from build123d import *

# Parameters (mm, degrees)
CROQUIS2_R                  = 4.1
SALIENTE_EXTRUIR1_DEPTH     = 35
CROQUIS3_W                  = 24
CROQUIS3_H                  = 12.1
CORTAR_EXTRUIR1_DEPTH       = 24
CROQUIS9_R                  = 1.7
CORTAR_EXTRUIR2_DEPTH       = 10
CORTAR_EXTRUIR3_START       = -10
CROQUIS11_R                 = 25
CORTAR_EXTRUIR3_DEPTH       = 10
CORTAR_EXTRUIR5_START       = 13.655231177
CORTAR_EXTRUIR5_DEPTH       = 8
CORTAR_EXTRUIR5_START_2     = 6.155231177
CORTAR_EXTRUIR5_2_DEPTH     = 5
CORTAR_EXTRUIR5_START_3     = 24.155231177
CORTAR_EXTRUIR5_3_DEPTH     = 5
CORTAR_EXTRUIR6_START       = -10
CROQUIS13_R                 = 25
CORTAR_EXTRUIR6_DEPTH       = 10
CROQUIS14_R                 = 11.035
CORTAR_EXTRUIR7_DEPTH       = 8.05
CORTAR_EXTRUIR8_DEPTH       = 15
CORTAR_EXTRUIR8_DEPTH_BACK  = 7
CORTAR_EXTRUIR9_DEPTH       = 15
CORTAR_EXTRUIR9_DEPTH_BACK  = 7
CORTAR_EXTRUIR10_DEPTH      = 15
CORTAR_EXTRUIR10_DEPTH_BACK = 7
CORTAR_EXTRUIR11_DEPTH      = 121.441894704
REDONDEO1_R                 = 30
CROQUIS22_W                 = 11.434183309
CROQUIS22_H                 = 8.348024574
CORTAR_EXTRUIR12_DEPTH      = 10


# Read off the part's stored shape, not the designer's step: Cortar-Extruir5
with BuildPart() as part:
    # Croquis2 → Saliente-Extruir1 (new body)
    with BuildSketch(Plane.XY):
        with BuildLine():
            Line((-11.5, 104.898979486), (-21.7, 104.898979486))
            Line((-21.7, 104.898979486), (-21.7, 100.380604651))
            Line((-21.7, 100.380604651), (-12.49420426, 100.380604651))
            ThreePointArc((-12.49420426, 100.380604651), (-12.498149406, 99.784915281), (-12.473709842, 99.189714392))
            ThreePointArc((-12.473709842, 99.189714392), (-16.573234399, 52.954310766), (-23.961892015, 7.129356989))
            ThreePointArc((-23.961892015, 7.129356989), (0, -25), (23.961892015, 7.129356989))
            ThreePointArc((23.961892015, 7.129356989), (16.547311175, 52.357383104), (12.33822575, 97.995458822))
            ThreePointArc((12.33822575, 97.995458822), (12.473356614, 99.184294915), (12.49420426, 100.380604651))
            Line((12.49420426, 100.380604651), (21.7, 100.380604651))
            Line((21.7, 100.380604651), (21.7, 104.898979486))
            Line((21.7, 104.898979486), (11.5, 104.898979486))
            ThreePointArc((11.5, 104.898979486), (0, 112.5), (-11.5, 104.898979486))
        make_face()
        Circle(CROQUIS2_R, mode=Mode.SUBTRACT)
    extrude(amount=SALIENTE_EXTRUIR1_DEPTH)

    # Croquis3 → Cortar-Extruir1 (cut)
    with BuildSketch(Plane(origin=(0, 112.5, 0), x_dir=(1, 0, 0), z_dir=(0, 1, 0))):
        with Locations((0, -17.5)):
            Rectangle(CROQUIS3_W, CROQUIS3_H)
    extrude(amount=-CORTAR_EXTRUIR1_DEPTH, mode=Mode.SUBTRACT)

    # Croquis9 → Cortar-Extruir2 (cut)
    with BuildSketch(Plane(origin=(0, 104.898979486, 0), x_dir=(1, 0, 0), z_dir=(0, 1, 0))):
        with Locations(Location((-15.2, -17.5, 0), (0, 0, 270))):
            Circle(CROQUIS9_R)
        with Locations(Location((15.2, -17.5, 0), (0, 0, 270))):
            Circle(CROQUIS9_R)
    extrude(amount=-CORTAR_EXTRUIR2_DEPTH, mode=Mode.SUBTRACT)

    # Croquis11 → Cortar-Extruir3 (cut)
    with BuildSketch(Plane.XY.offset(35).offset(CORTAR_EXTRUIR3_START)):
        Circle(CROQUIS11_R)
    extrude(amount=CORTAR_EXTRUIR3_DEPTH, mode=Mode.SUBTRACT)

    # Cortar-Extruir5 outline → Cortar-Extruir5 (cut)
    with BuildSketch(Plane.XY.offset(CORTAR_EXTRUIR5_START)):
        with BuildLine():
            Line((12.387970466, 97.129356989), (12, 97.129356989))
            Line((12, 97.129356989), (12, 88.5))
            Line((12, 88.5), (7.946995801, 88.5))
            ThreePointArc((7.946995801, 88.5), (12.16824242, 47.640569315), (18.961892015, 7.129356989))
            Line((18.961892015, 7.129356989), (23.961892015, 7.129356989))
            ThreePointArc((23.961892015, 7.129356989), (16.602493766, 51.9271429), (12.387970466, 97.129356989))
        make_face()
    extrude(amount=CORTAR_EXTRUIR5_DEPTH, mode=Mode.SUBTRACT)

    # Cortar-Extruir5 2 outline → Cortar-Extruir5 2 (cut)
    with BuildSketch(Plane.XY.offset(CORTAR_EXTRUIR5_START_2)):
        with BuildLine():
            ThreePointArc((12.902326037, 89.129356989), (12.63281503, 93.128564031), (12.387970466, 97.129356989))
            Line((12.387970466, 97.129356989), (7.387970466, 97.129356989))
            ThreePointArc((7.387970466, 97.129356989), (7.63281503, 93.128564031), (7.902326037, 89.129356989))
            Line((7.902326037, 89.129356989), (12.902326037, 89.129356989))
        make_face()
        with BuildLine():
            ThreePointArc((15.954808066, 57.129356989), (15.485901101, 61.127943182), (15.041769556, 65.129356989))
            Line((15.041769556, 65.129356989), (10.041769556, 65.129356989))
            ThreePointArc((10.041769556, 65.129356989), (10.485901101, 61.127943182), (10.954808066, 57.129356989))
            Line((10.954808066, 57.129356989), (15.954808066, 57.129356989))
        make_face()
        with BuildLine():
            ThreePointArc((18.985918027, 35.129356989), (18.378022509, 39.127504621), (17.795013863, 43.129356989))
            Line((17.795013863, 43.129356989), (12.795013863, 43.129356989))
            ThreePointArc((12.795013863, 43.129356989), (13.378022509, 39.127504621), (13.985918027, 35.129356989))
            Line((13.985918027, 35.129356989), (18.985918027, 35.129356989))
        make_face()
    extrude(amount=CORTAR_EXTRUIR5_2_DEPTH, mode=Mode.SUBTRACT)

    # Cortar-Extruir5 3 outline → Cortar-Extruir5 3 (cut)
    with BuildSketch(Plane.XY.offset(CORTAR_EXTRUIR5_START_3)):
        with BuildLine():
            ThreePointArc((13.684802762, 79.129356989), (13.35325681, 83.128371707), (13.046404729, 87.129356989))
            Line((13.046404729, 87.129356989), (8.046404729, 87.129356989))
            ThreePointArc((8.046404729, 87.129356989), (8.35325681, 83.128371707), (8.684802762, 79.129356989))
            Line((8.684802762, 79.129356989), (13.684802762, 79.129356989))
        make_face()
        with BuildLine():
            ThreePointArc((15.954808066, 57.129356989), (15.485901101, 61.127943182), (15.041769556, 65.129356989))
            Line((15.041769556, 65.129356989), (10.041769556, 65.129356989))
            ThreePointArc((10.041769556, 65.129356989), (10.485901101, 61.127943182), (10.954808066, 57.129356989))
            Line((10.954808066, 57.129356989), (15.954808066, 57.129356989))
        make_face()
        with BuildLine():
            ThreePointArc((18.985918027, 35.129356989), (18.378022509, 39.127504621), (17.795013863, 43.129356989))
            Line((17.795013863, 43.129356989), (12.795013863, 43.129356989))
            ThreePointArc((12.795013863, 43.129356989), (13.378022509, 39.127504621), (13.985918027, 35.129356989))
            Line((13.985918027, 35.129356989), (18.985918027, 35.129356989))
        make_face()
    extrude(amount=CORTAR_EXTRUIR5_3_DEPTH, mode=Mode.SUBTRACT)

    # Croquis13 → Cortar-Extruir6 (cut)
    with BuildSketch(Plane.XY.offset(25).offset(CORTAR_EXTRUIR6_START)):
        Circle(CROQUIS13_R)
    extrude(amount=CORTAR_EXTRUIR6_DEPTH, mode=Mode.SUBTRACT)

    # Croquis14 → Cortar-Extruir7 (cut)
    with BuildSketch(Plane(origin=(0, 0, 0), x_dir=(-1, 0, 0), z_dir=(0, 0, -1))):
        Circle(CROQUIS14_R)
    extrude(amount=-CORTAR_EXTRUIR7_DEPTH, mode=Mode.SUBTRACT)

    # Croquis16 → Cortar-Extruir8 (cut, two sides: drawn at the far end of the back side and taken through both)
    with BuildSketch(Plane(origin=(0, 0, 21.655231177), x_dir=(-1, 0, 0), z_dir=(0, 0, -1)).offset(-CORTAR_EXTRUIR8_DEPTH_BACK)):
        with BuildLine():
            Line((-13.627629456, 65.129356989), (-11.127629456, 65.129356989))
            ThreePointArc((-11.127629456, 65.129356989), (-11.671619883, 61.130083418), (-12.204820334, 57.129356989))
            Line((-12.204820334, 57.129356989), (-14.704820334, 57.129356989))
            ThreePointArc((-14.704820334, 57.129356989), (-14.1517613, 61.127409483), (-13.627629456, 65.129356989))
        make_face()
    extrude(amount=CORTAR_EXTRUIR8_DEPTH + CORTAR_EXTRUIR8_DEPTH_BACK, mode=Mode.SUBTRACT)

    # Croquis17 → Cortar-Extruir9 (cut, two sides: drawn at the far end of the back side and taken through both)
    with BuildSketch(Plane(origin=(0, 0, 21.655231177), x_dir=(-1, 0, 0), z_dir=(0, 0, -1)).offset(-CORTAR_EXTRUIR9_DEPTH_BACK)):
        with BuildLine():
            Line((-11.915557759, 97.129356989), (-9.415557759, 97.129356989))
            ThreePointArc((-9.415557759, 97.129356989), (-9.298046866, 93.126118397), (-9.554223154, 89.129356989))
            Line((-9.554223154, 89.129356989), (-12.054223154, 89.129356989))
            ThreePointArc((-12.054223154, 89.129356989), (-11.961814646, 93.128957012), (-11.915557759, 97.129356989))
        make_face()
    extrude(amount=CORTAR_EXTRUIR9_DEPTH + CORTAR_EXTRUIR9_DEPTH_BACK, mode=Mode.SUBTRACT)

    # Croquis18 → Cortar-Extruir10 (cut, two sides: drawn at the far end of the back side and taken through both)
    with BuildSketch(Plane(origin=(0, 0, 21.655231177), x_dir=(-1, 0, 0), z_dir=(0, 0, -1)).offset(-CORTAR_EXTRUIR10_DEPTH_BACK)):
        with BuildLine():
            Line((-16.345625555, 43.076723993), (-13.345625555, 43.076723993))
            ThreePointArc((-13.345625555, 43.076723993), (-13.91361536, 39.060592935), (-14.675658247, 35.076723993))
            Line((-14.675658247, 35.076723993), (-17.675658247, 35.076723993))
            ThreePointArc((-17.675658247, 35.076723993), (-16.863871756, 39.052322857), (-16.345625555, 43.076723993))
        make_face()
    extrude(amount=CORTAR_EXTRUIR10_DEPTH + CORTAR_EXTRUIR10_DEPTH_BACK, mode=Mode.SUBTRACT)

    # Croquis21 → Cortar-Extruir11 (cut, through all)
    with BuildSketch(Plane.XY.offset(35)):
        with BuildLine():
            Line((-12.473709842, 99.189714392), (-12.586604544, 52.126321873))
            ThreePointArc((-12.586604544, 52.126321873), (-15.474466118, 28.920051094), (-23.961892015, 7.129356989))
            Line((-23.961892015, 7.129356989), (-12.473709842, 99.189714392))
        make_face()
    extrude(amount=-CORTAR_EXTRUIR11_DEPTH, mode=Mode.SUBTRACT)

    # Redondeo1
    # the kernel refuses this fillet: 30 mm, written as the material it takes off along each edge
    with BuildSketch(Plane(origin=(-20.412546923, 14.433569486, 131.323871826), x_dir=(0.9503032831385696, 0.3113256655916044, 0), z_dir=(0, 0, -1))) as redondeo1_piece_1:
        with BuildLine():
            CenterArc((47.69462314, -24.085461873), REDONDEO1_R, 126.596996469, 71.521785283)
            ThreePointArc((19.182207947, -33.41510173), (11.30875316, -15.721520532), (0, 0))
            ThreePointArc((0, 0), (14.904569731, -4.928781773), (29.809139462, 0))
        make_face()
    extrude(amount=116.323871826, mode=Mode.SUBTRACT)

    # Croquis22 → Cortar-Extruir12 (cut)
    with BuildSketch(Plane(origin=(21.7, 0, 0), x_dir=(0, 0, -1), z_dir=(1, 0, 0))):
        with Locations((-17.832908346, 100.724967199)):
            Rectangle(CROQUIS22_W, CROQUIS22_H)
    extrude(amount=-CORTAR_EXTRUIR12_DEPTH, mode=Mode.SUBTRACT)


solid = part.part
Here's how the part is built. I have some questions about the finished solid (model axes, mm). A direction names the side the tool comes from. Coordinates: 2 decimals unless noted, no trailing zeros. Order: outer loops, then holes, each group sorted by start corner. A loop starts at its lowest first (then second) coordinate and runs counter-clockwise, first axis right, second up. Notation, with made-up numbers: M -32.75,32.5 L 12.25,32.5 A20 cw 12.25,43.5 Z; hole C 57,74.25 d7. An arc over 180 degrees is marked long. Answer as CSV lines item,"result".
Item 1: Imagine slicing it at D-D on z = 17.5. Write out the boundary of the cut face in (x, y), plus the area to 3 significant figures.
Results found:
outline,"M -21.7,100.38 L -16.9,100.38 L -16.9,104.9 L -21.7,104.9 Z; M -13.5,100.38 L -12.49,100.38 A12.5 ccw -12.47,99.19 L -12.59,52.13 A30 ccw 7.92,23.71 A25 cw 16.78,18.53 A650 cw 7.95,88.5 L -12,88.5 L -12,104.9 L -13.5,104.9 Z"
area,"1,440 mm2"
Item 2: Imagine slicing it at A-A on y = 0. Write out the boundary of the cut face in (x, z) (3 decimals), plus the area to 3 significant figures.
Results found:
outline,"M -25,0 L -11.035,0 L -11.035,8.05 L -4.1,8.05 L -4.1,15 L -25,15 Z; M 4.1,8.05 L 11.035,8.05 L 11.035,0 L 25,0 L 25,15 L 4.1,15 Z"
area,"515 mm2"
Item 3: We'd pull the mould along X, two halves only. Please class faces 4 (the face through (16, 39, 29.155)), 5 (the face through (0, -5, 8.05)), 6 (the face through (-6.762, 34.407, 25.14)): +X half, -X half, draft (parallel to the pull), parting line (faces both ways), or undercut.
Results found:
face 4,"draft"
face 5,"undercut"
face 6,"-X half"
Item 4: Imagine slicing it at C-C on y = 102.5. Write out the boundary of the cut face in (x, z), plus the area to 3 significant figures.
Results found:
outline,"M -21.7,0 L 21.7,0 L 21.7,12.12 L 12,12.12 L 12,11.45 L -12,11.45 L -12,23.55 L 21.7,23.55 L 21.7,35 L -21.7,35 Z; hole C -15.2,17.5 d3.4"
area,"1,110 mm2"
Item 5: For pin 1 (2 mm diameter, centred on y = 27, z = 14.5, fed in from -X); pin 2 (4 mm diameter, centred on x = -1, z = 30, fed in from -Y); pin 3 (3 mm diameter, centred on x = -17.5, z = 11.5, fed in from +Y), each with a flat end and sliding along its axis, tell me the tip position at first contact or that it passes through.
Results found:
pin 1,"x = -16.26"
pin 2,"y = 27.06"
pin 3,"y = 104.9"
Item 6: If I drill on line 1 (Z direction, x = 10.5, y = 62); line 2 (X direction, y = 0, z = 11.75); line 3 (X direction, y = 103.7, z = 17.5), over which ranges is the centre line in solid material (lowest first)?
Results found:
line 1,"0 to 6.16, 11.16 to 13.66, 21.66 to 24.16, 29.16 to 35"
line 2,"-25 to -4.1, 4.1 to 25"
line 3,"-21.7 to -16.9, -13.5 to -12"
Item 7: On a 3-axis mill with a long thin cutter (end or side, diameter ignored), from which of +Z, -Z, +X, -X, +Y, -Y can I reach the whole of each face in a straight line? I mean faces 1 (the face through (17, 104.899, 29)), 2 (the face through (-12, 97, 18)), 3 (the face through (15, 61, 11.155)). Say none if no direction works.
Results found:
face 1,"+Z, -Z, +X, +Y"
face 2,"+Y"
face 3,"+X"
Item 8: Imagine slicing it at B-B on z = 2. Write out the boundary of the cut face in (x, y) (3 decimals).
Results found:
outline,"M -23.962,7.129 A25 ccw long 23.962,7.129 A650 cw 12.338,97.995 A12.5 ccw 12.494,100.381 L 21.7,100.381 L 21.7,104.899 L 11.5,104.899 A12.5 ccw -11.5,104.899 L -21.7,104.899 L -21.7,100.381 L -12.494,100.381 A12.5 ccw -12.474,99.19 L -12.587,52.126 A94.684 cw Z; hole C 0,0 d22.07"
